Can you work these out from the model? Positions are in its coordinate system, mm. A direction names the side the tool comes from. Round coordinates to 2 decimals unless told otherwise and drop trailing zeros. Loops run counter-clockwise (first coordinate to the right, second up) from the corner with the lowest first, then second, coordinate; pieces in that order, holes last. Notation, with made-up numbers: (-9, 62.25) -> (2, 62.25) arc R13 ccw to (2, 85.25) -> close; hole circle Ø2 at (35, 33). An arc over 180 degrees is marked (long way). Use a Markdown table: item, result.
from build123d import *

# Parameters (mm, degrees)
F0_W     = 180
F0_H     = 31
F1_DEPTH = 25
F2_R     = 4
F3_DEPTH = 25.001
F4_W     = 4
F4_H     = 10.2
F5_DEPTH = 180.001


with BuildPart() as f1:
    # F0 (on Front) → F1 (new body)
    with BuildSketch(Plane.XZ):
        with Locations((90, 15.5)):
            Rectangle(F0_W, F0_H)
    extrude(amount=F1_DEPTH)

    # F2 (on face) → F3 (cut, through all)
    with BuildSketch(Plane(origin=(0, 0, 0), x_dir=(-1, 0, 0), z_dir=(0, 1, 0))):
        with Locations((-152, 26)):
            Circle(F2_R)
        with Locations((-48, 26)):
            Circle(F2_R)
    extrude(amount=-F3_DEPTH, mode=Mode.SUBTRACT)

    # F4 (on face) → F5 (cut, through all)
    with BuildSketch(Plane.YZ.offset(180)):
        with Locations((-23, 5.1)):
            Rectangle(F4_W, F4_H)
    extrude(amount=-F5_DEPTH, mode=Mode.SUBTRACT)


solid = f1.part
1. I want a section at A-A (x = 48). Please give me the cut outline in (y, z).
Answer sheet:
| item | result |
|---|---|
| outline | (-25, 10.2) -> (-21, 10.2) -> (-21, 0) -> (0, 0) -> (0, 22) -> (-25, 22) -> close; (-25, 30) -> (0, 30) -> (0, 31) -> (-25, 31) -> close |
2. I want a section at B-B (z = 26). Please give me the cut outline in (x, y).
Answer sheet:
| item | result |
|---|---|
| outline | (0, -25) -> (44, -25) -> (44, 0) -> (0, 0) -> close; (52, -25) -> (148, -25) -> (148, 0) -> (52, 0) -> close; (156, -25) -> (180, -25) -> (180, 0) -> (156, 0) -> close |
3. I want a section at D-D (x = 72.5). Please give me the cut outline in (y, z), plus the area to 3 significant figures.
Answer sheet:
| item | result |
|---|---|
| outline | (-25, 10.2) -> (-21, 10.2) -> (-21, 0) -> (0, 0) -> (0, 31) -> (-25, 31) -> close |
| area | 734 mm² |
4. If we mould it in two halves opening along X, with no side actions, what happens to faces 3 (the cylindrical face through (50.95, -12.32, 28.7)), 4 (the flat face through (180, -12, 15)), 5 (the flat face through (89, -10, 0))? For each: +X half, -X half, draft (parallel to the pull), parting line (faces both ways), or undercut.
Answer sheet:
| item | result |
|---|---|
| face 3 | undercut |
| face 4 | +X half |
| face 5 | draft |
5. I need wall thicknesses on line 1 (X direction, y = -5, z = 23.5); line 2 (X direction, y = -19.5, z = 24); line 3 (Z direction, x = 152, y = -15.75). Which ranges of each line are inside material? Lowest first, please.
Answer sheet:
| item | result |
|---|---|
| line 1 | x = 0 to 44.88, 51.12 to 148.88, 155.12 to 180 |
| line 2 | x = 0 to 44.54, 51.46 to 148.54, 155.46 to 180 |
| line 3 | z = 0 to 22, 30 to 31 |
6. Which directions (+Z, -Z, +X, -X, +Y, -Y) give clear straight access to the entire face, cutting with the end or side of a thin tool? Please do faces 1 (the flat face through (0, -12, 15)), 2 (the flat face through (91, -23, 10.2)).
Answer sheet:
| item | result |
|---|---|
| face 1 | +Z, -Z, -X, +Y, -Y |
| face 2 | -Z, +X, -X, -Y |
7. I want a section at C-C (y = -11.25). Please give me the cut outline in (x, z).
Answer sheet:
| item | result |
|---|---|
| outline | (0, 0) -> (180, 0) -> (180, 31) -> (0, 31) -> close; hole circle Ø8 at (48, 26); hole circle Ø8 at (152, 26) |
8. Will these pins go through, and if not, where does the flat tip stop? pin 1 Ø5 at (x, z) = (121.5, 6.5) entering from -Y; pin 2 Ø2 at (x, y) = (114.5, -23.5) entering from -Z.
Answer sheet:
| item | result |
|---|---|
| pin 1 | stops at y = -21 |
| pin 2 | stops at z = 10.2 |
